Geometry check sheet. Reference: drawing and pictorial views, mm from the part's lowest x, y, z. A direction names the side the tool comes from. Round coordinates to 2 decimals unless told otherwise and drop trailing zeros. Write each loop counter-clockwise with the first axis right and the second up, starting at its lowest first coordinate (ties: lowest second). Pieces come first, ordered by that corner, then holes. Notation, with made-up numbers: M -2,58 L 22,58 A10 ccw 22,70 Z; hole C 14,4.25 d8. An arc over 180 degrees is marked long. Answer in a Markdown table with one row per item.
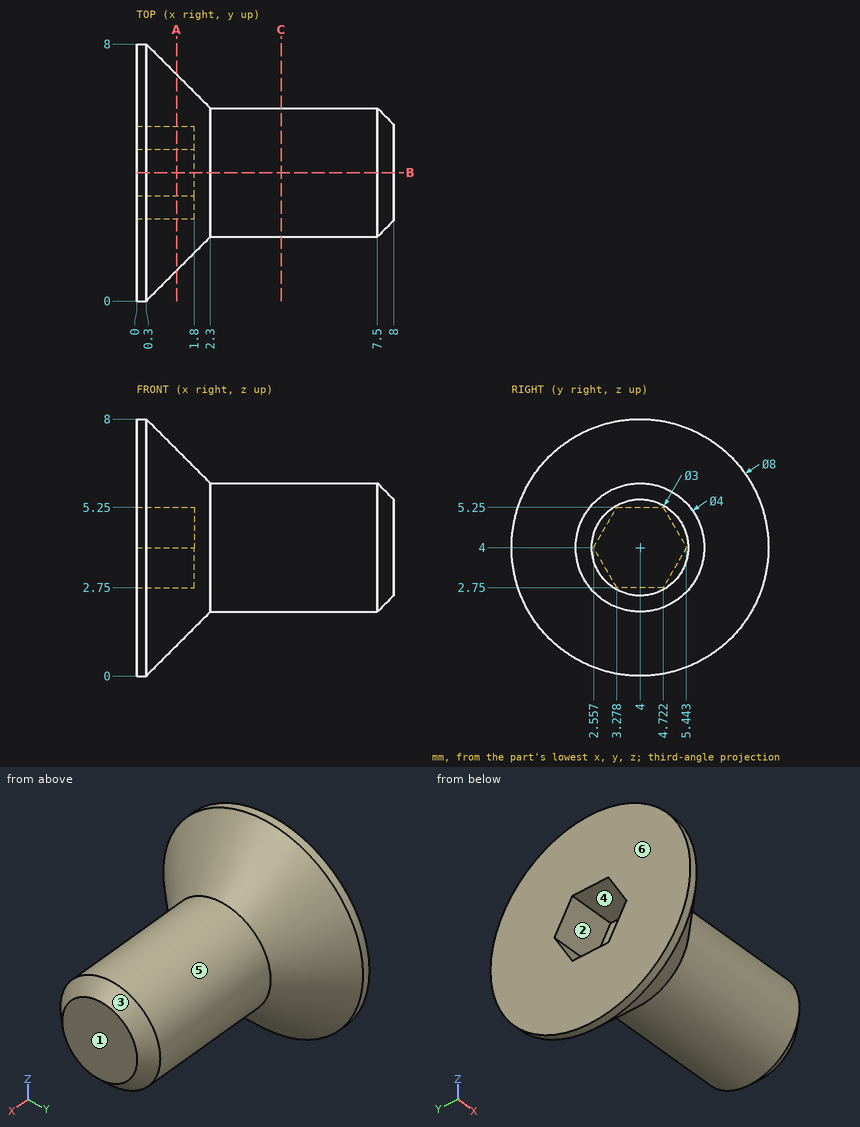
1. Access from +Z, -Z, +X, -X, +Y, -Y to the whole of each face (thin tool, end or side, straight path). Record for the marked faces 4, 5 and 6.
Found:
| item | result |
|---|---|
| face 4 | -X |
| face 5 | +X |
| face 6 | +Z, -Z, -X, +Y, -Y |
2. Scan lines: L1, parallel to Y at x = 1, z = 3.25 (1 decimal); L2, parallel to X at y = 4.75, z = 4.75; L3, parallel to X at y = 5.5, z = 7 (1 decimal). Record each from-to range of solid material in increasing order.
Found:
| item | result |
|---|---|
| L1 | y = 0.8 to 3, 5 to 7.2 |
| L2 | x = 1.8 to 8 |
| L3 | x = 0 to 0.9 |
3. Section check A-A, the plane x = 1.25. Record the cut outline in (y, z).
Found:
| item | result |
|---|---|
| outline | C 4,4 d6.1; hole M 2.56,4 L 3.28,2.75 L 4.72,2.75 L 5.44,4 L 4.72,5.25 L 3.28,5.25 Z |
4. Section check B-B, the plane y = 4. Record the cut outline in (x, z).
Found:
| item | result |
|---|---|
| outline | M 0,0 L 0.3,0 L 2.3,2 L 7.5,2 L 8,2.5 L 8,5.5 L 7.5,6 L 2.3,6 L 0.3,8 L 0,8 L 0,5.25 L 1.8,5.25 L 1.8,2.75 L 0,2.75 Z |
5. Draft check along Y on the marked faces 1, 2 and 3. Enter one of: +Y half, -Y half, draft (parallel to the pull), parting line (faces both ways), or undercut.
Found:
| item | result |
|---|---|
| face 1 | draft |
| face 2 | undercut |
| face 3 | parting line |
6. Section check C-C, the plane x = 4.5. Record the cut outline in (y, z).
Found:
| item | result |
|---|---|
| outline | C 4,4 d4 |
7. Go/stop test with flat-tipped pins: pin 1 (4 mm diameter, centred on x = 5.5, z = 1, fed in from +Y); pin 2 (0.8 mm diameter, centred on y = 4, z = 4, fed in from -X); pin 3 (1 mm diameter, centred on x = 1.5, y = 3.5, fed in from +Z). Record where each tip stops, or that it passes through.
Found:
| item | result |
|---|---|
| pin 1 | stops at y = 5.73 |
| pin 2 | stops at x = 1.8 |
| pin 3 | stops at z = 7.27 |
